Geometry: final body of the model. Coordinates: model frame, mm. Face numbers are marked on the shaded views. A direction names the side the tool comes from. Coordinates: 2 decimals unless noted, no trailing zeros. Loops run counter-clockwise (first coordinate to the right, second up) from the corner with the lowest first, then second, coordinate; pieces in that order, holes last. Notation, with made-up numbers: (30.5, 48) - (42.5, 48) arc R17 cw to (42.5, 56) - close; hole circle Ø8 at (-38, 45.5). An arc over 180 degrees is marked (long way). Return JSON: item names as keys, results as strings.
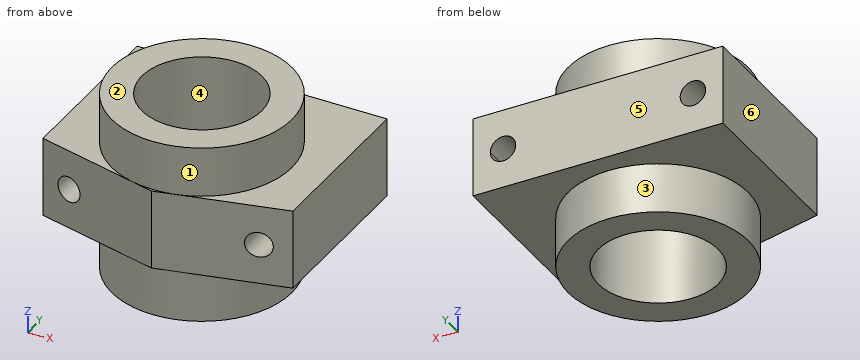
from build123d import *

# Parameters (mm, degrees)
SKETCH1_R               = 9.525
BOSS_EXTRUDE2_DEPTH     = 6.35
SKETCH2_R               = 14.2875
SKETCH2_R_2             = 9.525
BOSS_EXTRUDE3_DEPTH     = 14.2875
SKETCH6_R               = 2.0193
CUT_EXTRUDE1_DEPTH      = 17.4625
CUT_EXTRUDE2_DEPTH      = 31.047395504
CUT_EXTRUDE2_DEPTH_BACK = 31.047395504
SKETCH9_R               = 2.0193


with BuildPart() as part:
    # Sketch1 → Boss-Extrude2 (new, symmetric)
    with BuildSketch(Plane.XY):
        Polygon((19.84375, 0), (-19.84375, 0), (-19.84375, -17.4625), (-19.84375, -27.406149544), (0, -32.238619559), (19.84375, -27.406149544), (19.84375, -17.4625), align=None)
        with Locations((0, -17.533511157)):
            Circle(SKETCH1_R, mode=Mode.SUBTRACT)
    extrude(amount=BOSS_EXTRUDE2_DEPTH, both=True)

    # Sketch2 → Boss-Extrude3 (add, symmetric)
    with BuildSketch(Plane.XY):
        with Locations(Location((0, -17.533511157, 0), (0, 0, 180))):
            Circle(SKETCH2_R)
        with Locations((0, -17.533511157)):
            Circle(SKETCH2_R_2, mode=Mode.SUBTRACT)
    extrude(amount=BOSS_EXTRUDE3_DEPTH, both=True)

    # Sketch6 → Cut-Extrude1 (cut)
    with BuildSketch(Plane(origin=(0, 0, 0), x_dir=(1, 0, 0), z_dir=(0, 1, 0))):
        with Locations(Location((-15.08125, 0, 0), (0, 0, 270))):
            Circle(SKETCH6_R)
        with Locations(Location((15.08125, 0, 0), (0, 0, 90))):
            Circle(SKETCH6_R)
    extrude(amount=-CUT_EXTRUDE1_DEPTH, mode=Mode.SUBTRACT)

    # Sketch9 → Cut-Extrude2 (cut, two sides: drawn at the far end of the back side and taken through both)
    with BuildSketch(Plane(origin=(0, -17.4625, 0), x_dir=(1, 0, 0), z_dir=(0, 1, 0)).offset(-CUT_EXTRUDE2_DEPTH_BACK)):
        with Locations(Location((-15.08125, 0, 0), (0, 0, 270))):
            Circle(SKETCH9_R)
        with Locations((15.08125, 0)):
            Circle(SKETCH9_R)
    extrude(amount=CUT_EXTRUDE2_DEPTH + CUT_EXTRUDE2_DEPTH_BACK, mode=Mode.SUBTRACT)


solid = part.part
Item 1: First-contact query: pin 1 Ø6.5 at (x, z) = (15.08, 0) entering from -Y; pin 2 Ø3 at (y, z) = (-16.5, -10.5) entering from +X; pin 3 Ø3 at (x, z) = (-11.5, -4.5) entering from -Y. Flat tips, straight axial feed; report the tip coordinate or a pass-through.
Worked out:
{"pin 1": "y = -29.36", "pin 2": "x = 14.29", "pin 3": "y = -29.8"}
Item 2: Section query C-C, the plane x = 16. Return loops of the section in (y, z).
Worked out:
{"outline": "(-28.34, -6.35) - (0, -6.35) - (0, -1.8) - (-28.34, -1.8) - close; (-28.34, 1.8) - (0, 1.8) - (0, 6.35) - (-28.34, 6.35) - close"}
Item 3: Section query B-B, the plane z = 1. Return loops of the section in (x, y) (3 decimals).
Worked out:
{"outline": "(-19.844, -27.406) - (-16.836, -28.139) - (-16.836, 0) - (-19.844, 0) - close; (-13.327, -28.993) - (0, -32.239) - (13.327, -28.993) - (13.327, 0) - (-13.327, 0) - close; (16.836, -28.139) - (19.844, -27.406) - (19.844, 0) - (16.836, 0) - close; hole circle Ø19.05 at (0, -17.534)"}
Item 4: Section query A-A, the plane y = -14.5. Return loops of the section in (x, z).
Worked out:
{"outline": "(-19.84, -6.35) - (-13.96, -6.35) - (-13.96, -14.29) - (-9.03, -14.29) - (-9.03, 14.29) - (-13.96, 14.29) - (-13.96, 6.35) - (-19.84, 6.35) - close; (9.03, -14.29) - (13.96, -14.29) - (13.96, -6.35) - (19.84, -6.35) - (19.84, 6.35) - (13.96, 6.35) - (13.96, 14.29) - (9.03, 14.29) - close; hole circle Ø4.04 at (-15.08, 0); hole circle Ø4.04 at (15.08, 0)"}
Item 5: Section query D-D, the plane y = -2. Return loops of the section in (x, z), and give its area (3 significant figures).
Worked out:
{"outline": "(-19.84, -6.35) - (19.84, -6.35) - (19.84, 6.35) - (-19.84, 6.35) - close; hole circle Ø4.04 at (-15.08, 0); hole circle Ø4.04 at (15.08, 0)", "area": "478 mm^2"}
Item 6: Reachability of the marked faces 1, 2 and 3 from +Z, -Z, +X, -X, +Y, -Y: full face, straight path, thin tool, end or side. Return the list, or none.
Worked out:
{"face 1": "+Z", "face 2": "+Z, +X, -X, +Y, -Y", "face 3": "-Z"}
Item 7: Mould query, pull axis X, two halves, no side actions, for the marked faces 4, 5 and 6. Classes: +X half, -X half, draft (parallel to the pull), parting line (faces both ways), or undercut.
Worked out:
{"face 4": "undercut", "face 5": "draft", "face 6": "-X half"}
Item 8: Ray query, probe 1 along X at (y, z) = (-21.5, 0); probe 2 along Y at (x, z) = (7, -12.75); probe 3 along X at (y, z) = (-14.5, -5). Return the intervals inside material, ascending. Write a range as from..to.
Worked out:
{"probe 1": "-19.84..-17.1, -13.06..-8.66, 8.66..13.06, 17.1..19.84", "probe 2": "-29.99..-23.99, -11.07..-5.08", "probe 3": "-19.84..-9.03, 9.03..19.84"}
